Work out the finished part from the listing and answer in its coordinate system (mm). Coordinates: 2 decimals unless noted, no trailing zeros. Order: outer loops, then holes, each group sorted by start corner. A loop starts at its lowest first (then second) coordinate and runs counter-clockwise, first axis right, second up. Notation, with made-up numbers: M 15,4.25 L 74,4.25 A22 cw 74,43.25 Z; hole C -40,23 d2. An arc over 180 degrees is marked long. Use a Markdown table: item, result.
from build123d import *

# Parameters (mm, degrees)
F0_R     = 76.2
F0_R_2   = 3.175
F1_DEPTH = 1.5875
F3_DEPTH = 25.4


with BuildPart() as f1:
    # F0 (on Top) → F1 (new body)
    with BuildSketch(Plane.XY):
        Circle(F0_R)
        Circle(F0_R_2, mode=Mode.SUBTRACT)
    extrude(amount=F1_DEPTH)

    # F2 (on face) → F3 (cut)
    with BuildSketch(Plane.XY.offset(1.5875)):
        with BuildLine():
            Line((-25.4, 1.5875), (-69.85, 1.5875))
            ThreePointArc((-69.85, 1.5875), (-71.4375, 0), (-69.85, -1.5875))
            Line((-69.85, -1.5875), (-25.4, -1.5875))
            ThreePointArc((-25.4, -1.5875), (-23.8125, 0), (-25.4, 1.5875))
        make_face()
    extrude(amount=-F3_DEPTH, mode=Mode.SUBTRACT)


solid = f1.part
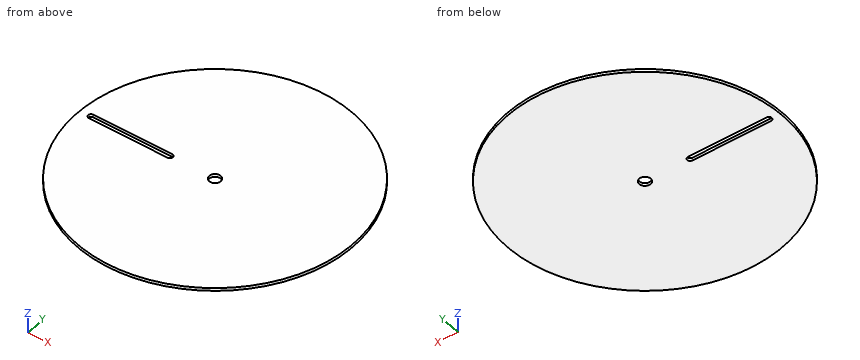
(1) A cutting plane is placed at B-B (z = 0.9). Give the number of separate pieces and of enclosed holes in the cut face, then the cut area to 3 significant figures.
Conclusion:
| item | result |
|---|---|
| separate pieces | 1 |
| enclosed holes | 2 |
| area | 18,100 mm2 |
(2) Straight lines are drawn through the part: L1, parallel to Y at x = 0, z = 0.55 (3 decimals); L2, parallel to Y at x = 47.5, z = 1.15; L3, parallel to Y at x = 10, z = 0.35. For each, find the intervals that lie inside material, in ascending order.
Conclusion:
| item | result |
|---|---|
| L1 | -76.2 to -3.175, 3.175 to 76.2 |
| L2 | -59.58 to 59.58 |
| L3 | -75.54 to 75.54 |
(3) A cutting plane is placed at C-C (x = -49). Determine the outline of the cut face in (y, z), then the cut area to 3 significant figures.
Conclusion:
| item | result |
|---|---|
| outline | M -58.36,0 L -1.59,0 L -1.59,1.59 L -58.36,1.59 Z; M 1.59,0 L 58.36,0 L 58.36,1.59 L 1.59,1.59 Z |
| area | 180 mm2 |
(4) A cutting plane is placed at D-D (y = 33). Determine the outline of the cut face in (x, z).
Conclusion:
| item | result |
|---|---|
| outline | M -68.68,0 L 68.68,0 L 68.68,1.59 L -68.68,1.59 Z |
(5) A cutting plane is placed at A-A (x = 0). Determine the outline of the cut face in (y, z) (1 decimal).
Conclusion:
| item | result |
|---|---|
| outline | M -76.2,0 L -3.2,0 L -3.2,1.6 L -76.2,1.6 Z; M 3.2,0 L 76.2,0 L 76.2,1.6 L 3.2,1.6 Z |
